Part model, mm, in its own coordinate system. Face numbers are marked on the shaded views. A direction names the side the tool comes from. Give positions to 0.01 mm unless a question says otherwise; leave off trailing zeros. Write each loop counter-clockwise with the first axis right and the second up, starting at its lowest first coordinate (ties: lowest second). Pieces come first, ordered by that corner, then holes. Notation, with made-up numbers: M 81.25,36.25 L 124.25,36.25 A18 cw 124.25,62.25 Z; hole C 10,27.5 d2. An arc over 180 degrees is marked long. Use a Markdown table: item, result.
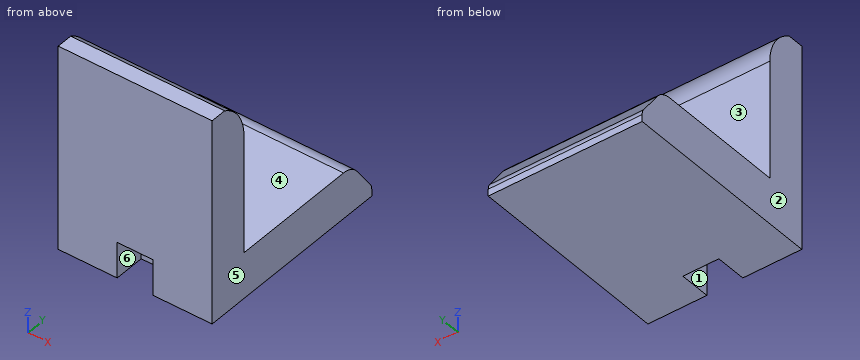
Solid Edge part; units mm, degrees
sketch "Sketch1" plane through (0, 0, 0) normal (-1, 0, 0) x (0, -1, 0)
  line L0 (-4, 4.5) -> (-4, 20)
  line L1 (-4, 20) -> (0, 20)
  line L2 (0, 20) -> (0, 0)
  line L3 (0, 0) -> (-20, 0)
  line L4 (-20, 0) -> (-20, 4.5)
  line L5 (-20, 4.5) -> (-4, 4.5)
extrude "Protrusion1" add sketch "Sketch1" along normal mid plane 15
sketch "Sketch2" plane through (0, 10, 0) normal (0, 0, -1) x (0, -1, 0)
  line L0 (10, -1.75) -> (7, -1.75)
  line L1 (10, 1.75) -> (10, -1.75)
  line L2 (10, 1.75) -> (7, 1.75)
  line L3 (7, -1.75) -> (7, 1.75)
extrude "ExtrudedCutout_1" cut sketch "Sketch2" against normal blind 3.5
chamfer "Chamfer_1" distance 2.5 distance2 3.5 1 edges at (0, 20, 4.5) measured on face at (-4.85, 17.4933, 4.5)
sketch "Sketch3" plane through (-7.5, 11, 10) normal (-1, 0, 0) x (0, -1, 0)
  line L0 (7, 6) -> (7, 10)
  line L1 (7, 10) -> (9.4384, 10)
  arc A0 (9.4384, 10) -> (7, 6) centre (11.5, 6) ccw
extrude "Cutout1" cut sketch "Sketch3" against normal through all
fillet "Round_1" radius 2 1 edges at (0, 17.5, 4.5)
fillet "Round_2" radius 1 1 edges at (0, 20, 1)
properties material "POM"
1. Drop flat-ended pins along their axis: P1, Ø9, axis at x = 1, z = 9.5, coming from the +Y side; P2, Ø3.5, axis at x = 1, y = 12, coming from the +Z side; P3, Ø1.5, axis at x = -0.5, y = 1.5, coming from the -Z side. Give the stop position or say it passes through.
Findings below:
| item | result |
|---|---|
| P1 | y = 4 |
| P2 | z = 4.5 |
| P3 | z = 3.5 |
2. Cut at B-B, the plane y = 11.25. Give the cut face in (x, z).
Findings below:
| item | result |
|---|---|
| outline | M -7.5,0 L 7.5,0 L 7.5,4.5 L -7.5,4.5 Z |
3. Cut at D-D, the plane x = 2.25. Give the cut face in (y, z).
Findings below:
| item | result |
|---|---|
| outline | M 0,0 L 20,0 L 20,0.68 A1 ccw 19.81,1.26 L 18.1,3.66 A2 ccw 16.47,4.5 L 4,4.5 L 4,16 A4.5 ccw 1.56,20 L 0,20 Z |
4. Tool access for the marked faces 1, 2 and 3: list every direction of +Z, -Z, +X, -X, +Y, -Y with a clear straight run to the whole face (end or side of a thin tool).
Findings below:
| item | result |
|---|---|
| face 1 | -Z, -Y |
| face 2 | +Z, -Z, -X, +Y, -Y |
| face 3 | +Z, +X, -X, +Y |
5. Two-plate mould, pull along X, no slides. Class the marked faces 4, 5 and 6: released by +X, released by -X, zero draft, split by the parting line, or undercut.
Findings below:
| item | result |
|---|---|
| face 4 | zero draft |
| face 5 | released by +X |
| face 6 | undercut |
6. Cut at C-C, the plane z = 12.25. Give the cut face in (x, y), then the cut area to 3 significant figures.
Findings below:
| item | result |
|---|---|
| outline | M -7.5,0 L 7.5,0 L 7.5,4 L -7.5,4 Z |
| area | 60.0 mm2 |
7. Drill centre lines: L1, parallel to Y at x = 1.75, z = 15.25; L2, parallel to Z at x = 4, y = 9.75; L3, parallel to Z at x = 6, y = 18.75. Where is each one in solid material? Low to high.
Findings below:
| item | result |
|---|---|
| L1 | 0 to 4 |
| L2 | 0 to 4.5 |
| L3 | 0 to 2.75 |
8. Cut at A-A, the plane x = 0.75. Give the cut face in (y, z), then the cut area to 3 significant figures.
Findings below:
| item | result |
|---|---|
| outline | M 0,3.5 L 3,3.5 L 3,0 L 20,0 L 20,0.68 A1 ccw 19.81,1.26 L 18.1,3.66 A2 ccw 16.47,4.5 L 4,4.5 L 4,16 A4.5 ccw 1.56,20 L 0,20 Z |
| area | 134 mm2 |
